```python
from build123d import *

# Parameters (mm, degrees)
SKETCH1_R            = 35.5
BOSS_EXTRUDE1_DEPTH  = 2
SKETCH2_R            = 35.5
SKETCH2_R_2          = 34
BOSS_EXTRUDE2_DEPTH  = 9.2
SKETCH5_R            = 34
SKETCH5_R_2          = 28.75
BOSS_EXTRUDE3_DEPTH  = 1.5
CUT_EXTRUDE2_REACH   = 53.439
CUT_EXTRUDE3_REACH   = 53.041
M2_CLEARANCE_HOLE1_D = 2.4
SKETCH10_R           = 1.2
CUT_EXTRUDE4_DEPTH   = 2.5


with BuildPart() as part:
    # Sketch1 → Boss-Extrude1 (new body)
    with BuildSketch(Plane.XZ):
        with Locations(Location((0, 0, 0), (0, 0, 270))):
            Circle(SKETCH1_R)
    extrude(amount=BOSS_EXTRUDE1_DEPTH)

    # Sketch2 → Boss-Extrude2 (add)
    with BuildSketch(Plane.XZ.offset(2)):
        with Locations(Location((0, 0, 0), (0, 0, 270))):
            Circle(SKETCH2_R)
        with Locations(Location((0, 0, 0), (0, 0, 270))):
            Circle(SKETCH2_R_2, mode=Mode.SUBTRACT)
    extrude(amount=BOSS_EXTRUDE2_DEPTH)

    # Sketch5 → Boss-Extrude3 (add)
    with BuildSketch(Plane.XZ.offset(2)):
        with Locations(Location((0, 0, 0), (0, 0, 270))):
            Circle(SKETCH5_R)
        with Locations(Location((0, 0, 0), (0, 0, 270))):
            Circle(SKETCH5_R_2, mode=Mode.SUBTRACT)
    extrude(amount=BOSS_EXTRUDE3_DEPTH)

    # Sketch3 → Cut-Extrude2 (cut, up to next)
    with BuildSketch(Plane(origin=(0, 0, 0), x_dir=(1, 0, 0), z_dir=(0, 1, 0)), mode=Mode.PRIVATE) as cut_extrude2_sk1:
        with BuildLine():
            Line((-17.298843892, 31), (17.298843892, 31))
            ThreePointArc((17.298843892, 31), (0, 35.5), (-17.298843892, 31))
        make_face()
    cut_extrude2_tool1 = extrude(cut_extrude2_sk1.sketch, amount=-CUT_EXTRUDE2_REACH, mode=Mode.PRIVATE) & part.part
    add(cut_extrude2_tool1.solids().sort_by_distance((0, 0, -32.810151))[0], mode=Mode.SUBTRACT)

    # Sketch6 → Cut-Extrude3 (cut, up to next)
    with BuildSketch(Plane.XZ.offset(2), mode=Mode.PRIVATE) as cut_extrude3_sk1:
        Polygon((-18.869547058, -31), (-16, -23.886450134), (16, -23.886450134), (18.869547058, -31), align=None)
    cut_extrude3_tool1 = extrude(cut_extrude3_sk1.sketch, amount=CUT_EXTRUDE3_REACH, mode=Mode.PRIVATE) & part.part
    add(cut_extrude3_tool1.solids().sort_by_distance((0, -2, -27.540792))[0], mode=Mode.SUBTRACT)

    # M2 Clearance Hole1 (through all)
    with Locations(Plane(origin=(0, 0, 0), x_dir=(1, 0, 0), z_dir=(0, 1, 0))):
        with Locations((-20.5, 23.916521486), (-31.5, 0), (-20.5, -23.916521486), (31.5, 0), (20.5, 23.916521486), (20.5, -23.916521486)):
            Hole(M2_CLEARANCE_HOLE1_D / 2)

    # Sketch10 → Cut-Extrude4 (cut)
    # profile 1 of 6: a face of its own
    with BuildSketch(Plane(origin=(0, 0, 0), x_dir=(1, 0, 0), z_dir=(0, 1, 0))):
        with BuildLine():
            Line((-35.446403203, 1.95), (-31.5, 1.95))
            ThreePointArc((-31.5, 1.95), (-29.55, 0), (-31.5, -1.95))
            Line((-31.5, -1.95), (-35.446403203, -1.95))
            ThreePointArc((-35.446403203, -1.95), (-35.5, 0), (-35.446403203, 1.95))
        make_face()
        with Locations(Location((-31.5, 0, 0), (0, 0, 270))):
            Circle(SKETCH10_R, mode=Mode.SUBTRACT)
    # profile 2 of 6: a face of its own
    with BuildSketch(Plane(origin=(0, 0, 0), x_dir=(1, 0, 0), z_dir=(0, 1, 0))):
        with BuildLine():
            Line((-24.548840716, 25.643798851), (-21.980546568, 22.647473867))
            ThreePointArc((-21.980546568, 22.647473867), (-19.230952381, 22.435974918), (-19.019453432, 25.185569105))
            Line((-19.019453432, 25.185569105), (-21.58774758, 28.181894089))
            ThreePointArc((-21.58774758, 28.181894089), (-23.103174603, 26.953540088), (-24.548840716, 25.643798851))
        make_face()
        with Locations(Location((-20.5, 23.916521486, 0), (0, 0, 270))):
            Circle(SKETCH10_R, mode=Mode.SUBTRACT)
    # profile 3 of 6: a face of its own
    with BuildSketch(Plane(origin=(0, 0, 0), x_dir=(1, 0, 0), z_dir=(0, 1, 0))):
        with BuildLine():
            Line((-21.58774758, -28.181894089), (-19.019453432, -25.185569105))
            ThreePointArc((-19.019453432, -25.185569105), (-19.230952381, -22.435974918), (-21.980546568, -22.647473867))
            Line((-21.980546568, -22.647473867), (-24.548840716, -25.643798851))
            ThreePointArc((-24.548840716, -25.643798851), (-23.103174603, -26.953540088), (-21.58774758, -28.181894089))
        make_face()
        with Locations(Location((-20.5, -23.916521486, 0), (0, 0, 270))):
            Circle(SKETCH10_R, mode=Mode.SUBTRACT)
    # profile 4 of 6: a face of its own
    with BuildSketch(Plane(origin=(0, 0, 0), x_dir=(1, 0, 0), z_dir=(0, 1, 0))):
        with BuildLine():
            Line((24.548840716, -25.643798851), (21.980546568, -22.647473867))
            ThreePointArc((21.980546568, -22.647473867), (19.230952381, -22.435974918), (19.019453432, -25.185569105))
            Line((19.019453432, -25.185569105), (21.58774758, -28.181894089))
            ThreePointArc((21.58774758, -28.181894089), (23.103174603, -26.953540088), (24.548840716, -25.643798851))
        make_face()
        with Locations(Location((20.5, -23.916521486, 0), (0, 0, 90))):
            Circle(SKETCH10_R, mode=Mode.SUBTRACT)
    # profile 5 of 6: a face of its own
    with BuildSketch(Plane(origin=(0, 0, 0), x_dir=(1, 0, 0), z_dir=(0, 1, 0))):
        with BuildLine():
            Line((21.58774758, 28.181894089), (19.019453432, 25.185569105))
            ThreePointArc((19.019453432, 25.185569105), (19.230952381, 22.435974918), (21.980546568, 22.647473867))
            Line((21.980546568, 22.647473867), (24.548840716, 25.643798851))
            ThreePointArc((24.548840716, 25.643798851), (23.103174603, 26.953540088), (21.58774758, 28.181894089))
        make_face()
        with Locations(Location((20.5, 23.916521486, 0), (0, 0, 90))):
            Circle(SKETCH10_R, mode=Mode.SUBTRACT)
    # profile 6 of 6: a face of its own
    with BuildSketch(Plane(origin=(0, 0, 0), x_dir=(1, 0, 0), z_dir=(0, 1, 0))):
        with BuildLine():
            Line((35.446403203, -1.95), (31.5, -1.95))
            ThreePointArc((31.5, -1.95), (29.55, 0), (31.5, 1.95))
            Line((31.5, 1.95), (35.446403203, 1.95))
            ThreePointArc((35.446403203, 1.95), (35.5, 0), (35.446403203, -1.95))
        make_face()
        with Locations(Location((31.5, 0, 0), (0, 0, 90))):
            Circle(SKETCH10_R, mode=Mode.SUBTRACT)
    extrude(amount=-CUT_EXTRUDE4_DEPTH, mode=Mode.SUBTRACT)


solid = part.part
```
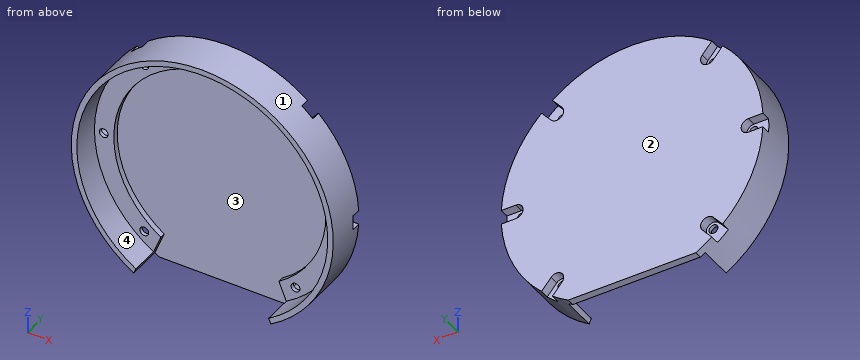
Part model, mm, in its own coordinate system. Face numbers are marked on the shaded views. Give positions to 0.01 mm unless a question says otherwise; leave off trailing zeros. Order: outer loops, then holes, each group sorted by start corner. A loop starts at its lowest first (then second) coordinate and runs counter-clockwise, first axis right, second up. Notation, with made-up numbers: M 82.5,69 L 119.5,69 A10 cw 119.5,75 Z; hole C 31,29.5 d7. An arc over 180 degrees is marked long. Use a Markdown table: item, result. Add a question column.
(1) Saw through at B-B, the plane x = 0. Give the cut face in (y, z), and give its area (3 significant figures).
(2) Saw through at C-C, the plane y = -1. Give the cut face in (x, z).
(3) Probe line 1 along Z through (x, y) = (-20, -0.5); line 2 along Z through (x, y) = (-20.5, -2.9); line 3 along Y through (x, z) = (-20.5, -21). List the from-to ranges inside material, lowest first. Write a range as [from, to].
(4) Saw through at D-D, the plane x = -20.5. Give the cut face in (y, z).
(5) Saw through at A-A, the plane z = 0. Give the cut face in (x, y).
(6) Drop flat-ended pins along their axis: P1, Ø6, axis at x = 26.5, y = -6, coming from the -Z side; P2, Ø1.8, axis at x = 20.5, z = 24, coming from the +Y side (1 decimal); P3, Ø1, axis at x = -3.5, z = 7, coming from the +Y side; P4, Ø1, axis at y = -6, z = -18.5, coming from the -X side. Give the stop position or say it passes through.
(7) Mould opens along Z. For the marked faces 1, 2, 3 and 4 say: +Z half, -Z half, draft (parallel to the pull), parting line (faces both ways), or undercut.
Answer key:
| question | item | result |
|---|---|---|
| 1 | outline | M -11.2,34 L -3.5,34 L -3.5,28.75 L -2,28.75 L -2,-31 L 0,-31 L 0,35.5 L -11.2,35.5 Z |
| 1 | area | 155 mm^2 |
| 2 | outline | M -35.45,-1.95 A35.5 ccw -24.55,-25.64 L -21.98,-22.65 A1.95 cw -19.02,-25.19 L -21.59,-28.18 A35.5 ccw -17.3,-31 L 17.3,-31 A35.5 ccw 21.59,-28.18 L 19.02,-25.19 A1.95 cw 21.98,-22.65 L 24.55,-25.64 A35.5 ccw 35.45,-1.95 L 31.5,-1.95 A1.95 cw 31.5,1.95 L 35.45,1.95 A35.5 ccw 24.55,25.64 L 21.98,22.65 A1.95 cw 19.02,25.19 L 21.59,28.18 A35.5 ccw -21.59,28.18 L -19.02,25.19 A1.95 cw -21.98,22.65 L -24.55,25.64 A35.5 ccw -35.45,1.95 L -31.5,1.95 A1.95 cw -31.5,-1.95 Z |
| 3 | line 1 | [-29.33, -26.33], [-22.03, 22.03], [26.33, 29.33] |
| 3 | line 2 | [-28.98, -25.12], [-22.72, -20.16], [20.16, 22.72], [25.12, 28.98] |
| 3 | line 3 | [-3.5, 0] |
| 4 | outline | M -11.2,-28.98 L 0,-28.98 L 0,-26.91 L -2.5,-26.91 L -2.5,-25.12 L -3.5,-25.12 L -3.5,-27.12 L -11.2,-27.12 Z; M -11.2,27.12 L -3.5,27.12 L -3.5,25.12 L -2.5,25.12 L -2.5,26.91 L 0,26.91 L 0,28.98 L -11.2,28.98 Z; M -3.5,-22.72 L -2.5,-22.72 L -2.5,-21.97 L 0,-21.97 L 0,21.97 L -2.5,21.97 L -2.5,22.72 L -3.5,22.72 L -3.5,20.16 L -2,20.16 L -2,-20.16 L -3.5,-20.16 Z |
| 5 | outline | M -35.5,-11.2 L -34,-11.2 L -34,-3.5 L -32.7,-3.5 L -32.7,-2.5 L -35.5,-2.5 Z; M -30.3,-3.5 L -28.75,-3.5 L -28.75,-2 L 28.75,-2 L 28.75,-3.5 L 30.3,-3.5 L 30.3,-2.5 L 29.55,-2.5 L 29.55,0 L -29.55,0 L -29.55,-2.5 L -30.3,-2.5 Z; M 32.7,-3.5 L 34,-3.5 L 34,-11.2 L 35.5,-11.2 L 35.5,-2.5 L 32.7,-2.5 Z |
| 6 | P1 | z = -26.61 |
| 6 | P2 | through |
| 6 | P3 | y = 0 |
| 6 | P4 | x = -30.6 |
| 7 | face 1 | parting line |
| 7 | face 2 | draft |
| 7 | face 3 | undercut |
| 7 | face 4 | undercut |
